```python
from build123d import *

# Parameters (mm, degrees)
SKETCH1_W                      = 55
SKETCH1_H                      = 55
BOSS_EXTRUDE1_DEPTH            = 6.35
SKETCH2_W                      = 11.25
SKETCH2_H                      = 11.25
CUT_EXTRUDE1_DEPTH             = 40.405868852
SKETCH3_W                      = 14
SKETCH3_H                      = 8.5
CUT_EXTRUDE2_DEPTH             = 2
CBORE_FOR_M2_SHCS2_D           = 2.4
CBORE_FOR_M2_SHCS2_CBORE_D     = 4.4
CBORE_FOR_M2_SHCS2_CBORE_DEPTH = 2
SKETCH6_R                      = 4
BOSS_EXTRUDE2_DEPTH            = 9.5
CBORE_FOR_M2_SHCS1_D           = 2.4
CBORE_FOR_M2_SHCS1_CBORE_D     = 4.4
CBORE_FOR_M2_SHCS1_CBORE_DEPTH = 2
SKETCH13_R                     = 3.025
CUT_EXTRUDE4_DEPTH             = 1
CHAMFER1_SIZE                  = 1.75
SKETCH16_W                     = 10
SKETCH16_H                     = 10
BOSS_EXTRUDE3_DEPTH            = 6.35
SKETCH17_R                     = 2.55
CUT_EXTRUDE6_DEPTH             = 50.129649907
FILLET1_R                      = 5
FILLET2_R                      = 1
SKETCH18_R                     = 3.025
CUT_EXTRUDE7_DEPTH             = 1
CUT_EXTRUDE8_DEPTH             = 0.6
CHAMFER2_SIZE                  = 1.5


with BuildPart() as part:
    # Sketch1 → Boss-Extrude1 (new body)
    with BuildSketch(Plane(origin=(0, 0, 0), x_dir=(1, 0, 0), z_dir=(0, 1, 0))):
        Rectangle(SKETCH1_W, SKETCH1_H)
    extrude(amount=BOSS_EXTRUDE1_DEPTH)

    # Sketch2 → Cut-Extrude1 (cut, through all)
    with BuildSketch(Plane(origin=(0, 6.35, 0), x_dir=(1, 0, 0), z_dir=(0, 1, 0))):
        Rectangle(SKETCH2_W, SKETCH2_H)
    extrude(amount=-CUT_EXTRUDE1_DEPTH, mode=Mode.SUBTRACT)

    # Sketch3 → Cut-Extrude2 (cut)
    with BuildSketch(Plane(origin=(0, 6.35, 0), x_dir=(1, 0, 0), z_dir=(0, 1, 0))):
        with Locations((0, -9.875)):
            Rectangle(SKETCH3_W, SKETCH3_H)
    extrude(amount=-CUT_EXTRUDE2_DEPTH, mode=Mode.SUBTRACT)

    # CBORE for M2 SHCS2 (through all)
    with Locations(Plane.XZ):
        with Locations((10.5, -0.1), (10.5, 12.4), (-10.5, 12.4), (-10.5, -0.1)):
            CounterBoreHole(CBORE_FOR_M2_SHCS2_D / 2, CBORE_FOR_M2_SHCS2_CBORE_D / 2, CBORE_FOR_M2_SHCS2_CBORE_DEPTH)

    # Sketch6 → Boss-Extrude2 (add)
    with BuildSketch(Plane(origin=(0, 6.35, 0), x_dir=(1, 0, 0), z_dir=(0, 1, 0))):
        with Locations(Location((-20, 20, 0), (0, 0, 270))):
            Circle(SKETCH6_R)
        with Locations(Location((20, 20, 0), (0, 0, 270))):
            Circle(SKETCH6_R)
        with Locations(Location((20, -20, 0), (0, 0, 270))):
            Circle(SKETCH6_R)
        with Locations(Location((-20, -20, 0), (0, 0, 270))):
            Circle(SKETCH6_R)
    extrude(amount=BOSS_EXTRUDE2_DEPTH)

    # CBORE for M2 SHCS1 (through all)
    with Locations(Plane.XZ):
        with Locations((-20, -20), (-20, 20), (20, 20), (20, -20)):
            CounterBoreHole(CBORE_FOR_M2_SHCS1_D / 2, CBORE_FOR_M2_SHCS1_CBORE_D / 2, CBORE_FOR_M2_SHCS1_CBORE_DEPTH)

    # Sketch13 → Cut-Extrude4 (cut)
    with BuildSketch(Plane(origin=(0, 6.35, 0), x_dir=(1, 0, 0), z_dir=(0, 1, 0))):
        with Locations(Location((-10.5, -12.4, 0), (0, 0, 270))):
            Circle(SKETCH13_R)
        with Locations(Location((-10.5, 0.1, 0), (0, 0, 270))):
            Circle(SKETCH13_R)
        with Locations(Location((10.5, -12.4, 0), (0, 0, 90))):
            Circle(SKETCH13_R)
        with Locations(Location((10.5, 0.1, 0), (0, 0, 90))):
            Circle(SKETCH13_R)
    extrude(amount=-CUT_EXTRUDE4_DEPTH, mode=Mode.SUBTRACT)

    # Chamfer1
    chamfer1_edges = [part.edges().sort_by_distance(p)[0] for p in [
        (5.625, 0, 0),
        (0, 0, 5.625),
        (-5.625, 0, 0),
        (0, 0, -5.625),
    ]]
    chamfer(chamfer1_edges, length=CHAMFER1_SIZE)

    # Sketch16 → Boss-Extrude3 (add)
    with BuildSketch(Plane.XZ):
        with Locations((32.5, 0)):
            Rectangle(SKETCH16_W, SKETCH16_H)
        with Locations((-32.5, 0)):
            Rectangle(SKETCH16_W, SKETCH16_H)
    extrude(amount=-BOSS_EXTRUDE3_DEPTH)

    # Sketch17 → Cut-Extrude6 (cut, through all)
    with BuildSketch(Plane.XZ):
        with Locations(Location((32.5, 0, 0), (0, 0, 270))):
            Circle(SKETCH17_R)
        with Locations(Location((-32.5, 0, 0), (0, 0, 270))):
            Circle(SKETCH17_R)
    extrude(amount=-CUT_EXTRUDE6_DEPTH, mode=Mode.SUBTRACT)

    # Fillet1
    fillet1_edges = [part.edges().sort_by_distance(p)[0] for p in [
        (27.5, 3.175, 5),
        (27.5, 3.175, -5),
        (-27.5, 3.175, -5),
        (-27.5, 3.175, 5),
        (27.5, 3.175, 27.5),
        (-27.5, 3.175, 27.5),
        (-27.5, 3.175, -27.5),
        (27.5, 3.175, -27.5),
    ]]
    fillet(fillet1_edges, radius=FILLET1_R)

    # Fillet2
    fillet2_edges = [part.edges().sort_by_distance(p)[0] for p in [
        (37.5, 3.175, -5),
        (37.5, 3.175, 5),
        (-37.5, 3.175, 5),
        (-37.5, 3.175, -5),
    ]]
    fillet(fillet2_edges, radius=FILLET2_R)

    # Sketch18 → Cut-Extrude7 (cut)
    with BuildSketch(Plane(origin=(0, 15.85, 0), x_dir=(1, 0, 0), z_dir=(0, 1, 0))):
        with Locations(Location((-20, 20, 0), (0, 0, 270))):
            Circle(SKETCH18_R)
        with Locations(Location((-20, -20, 0), (0, 0, 270))):
            Circle(SKETCH18_R)
        with Locations(Location((20, 20, 0), (0, 0, 270))):
            Circle(SKETCH18_R)
        with Locations(Location((20, -20, 0), (0, 0, 270))):
            Circle(SKETCH18_R)
    extrude(amount=-CUT_EXTRUDE7_DEPTH, mode=Mode.SUBTRACT)

    # Sketch19 → Cut-Extrude8 (cut)
    with BuildSketch(Plane(origin=(0, 6.35, 0), x_dir=(1, 0, 0), z_dir=(0, 1, 0))):
        Polygon((-2.301535791, 15.658119658), (-3.093589744, 15.658119658), (-3.093589744, 18.426068376), (-3.473504274, 18.426068376), (-3.473504274, 19.131623932), (-3.093589744, 19.131623932), (-3.093589744, 20), (-2.333760684, 20), (-2.333760684, 19.131623932), (-0.542735043, 19.131623932), (-0.542735043, 18.362466613), align=None)
        Polygon((-2.333760684, 18.426068376), (-2.333760684, 16.985276442), (-1.396694712, 18.426068376), align=None, mode=Mode.SUBTRACT)
        Polygon((3.55491453, 15.766666667), (2.743356036, 15.766666667), (1.65534188, 18.773758013), (0.564783654, 15.766666667), (-0.244230769, 15.766666667), (1.290691774, 20), (2.022536058, 20), align=None)
    extrude(amount=-CUT_EXTRUDE8_DEPTH, mode=Mode.SUBTRACT)

    # Chamfer2
    chamfer2_edges = [part.edges().sort_by_distance(p)[0] for p in [
        (-20, 6.35, -24),
        (20, 6.35, -24),
        (20, 6.35, 16),
        (-20, 6.35, 16),
    ]]
    chamfer(chamfer2_edges, length=CHAMFER2_SIZE)


solid = part.part
```
Verification items for the finished model (mm, model axes). A direction names the side the tool comes from. Round coordinates to 2 decimals unless told otherwise and drop trailing zeros. Write each loop counter-clockwise with the first axis right and the second up, starting at its lowest first coordinate (ties: lowest second). Pieces come first, ordered by that corner, then holes. Notation, with made-up numbers: (-28.75, 21.5) -> (-2.75, 21.5) arc R5 ccw to (-2.75, 27.5) -> close; hole circle Ø2 at (6, 75.5). An arc over 180 degrees is marked (long way). Write each question's results on one line, items separated by ' | '.
Q1. Sectioned sample at B-B, the plane z = 12.4. Give the number of separate pieces and of enclosed holes in the cut face, and give its area (3 significant figures).
Derived:
separate pieces: 3 | enclosed holes: 0 | area: 275 mm²
Q2. Sectioned sample at C-C, the plane x = -31. Record the boundary of the cut face in (y, z), and give its area (3 significant figures).
Derived:
outline: (0, -5.23) -> (6.35, -5.23) -> (6.35, -2.06) -> (0, -2.06) -> close; (0, 2.06) -> (6.35, 2.06) -> (6.35, 5.23) -> (0, 5.23) -> close | area: 40.2 mm²
Q3. Draft check along X on faces 1 (the face through (20.26, 8.51, -21.17)), 2 (the face through (-29, 3.22, -6.43)), 3 (the face through (27.5, 3, 16)). Enter one of: released by +X, released by -X, zero draft, split by the parting line, or undercut.
Derived:
face 1: undercut | face 2: released by -X | face 3: released by +X
Q4. Thickness scan on probe 1 along Z at (x, y) = (20, 1.05); probe 2 along X at (y, z) = (1.5, 21.5); probe 3 along Z at (x, y) = (-9, 5.5). Record the ranges inside material, lowest first.
Derived:
probe 1: z = -27.5 to -22.2, -17.8 to 17.8, 22.2 to 27.5 | probe 2: x = -27.5 to -21.61, -18.39 to 18.39, 21.61 to 27.5 | probe 3: z = -27.5 to -2.73, 2.53 to 9.77, 15.03 to 27.5
Q5. Sectioned sample at A-A, the plane y = 12. Record the boundary of the cut face in (x, z), and give its area (3 significant figures).
Derived:
outline: circle Ø8 at (-20, -20); circle Ø8 at (-20, 20); circle Ø8 at (20, -20); circle Ø8 at (20, 20); hole circle Ø2.4 at (-20, -20); hole circle Ø2.4 at (-20, 20); hole circle Ø2.4 at (20, -20); hole circle Ø2.4 at (20, 20) | area: 183 mm²
Q6. Access from +Z, -Z, +X, -X, +Y, -Y to the whole of each face (thin tool, end or side, straight path). Record for faces 4 (the face through (0, 3, 5.625)), 5 (the face through (27.5, 3, -16)), 6 (the face through (-27.5, 3, -16)).
Derived:
face 4: +Y, -Y | face 5: -Z, +X, +Y, -Y | face 6: -Z, -X, +Y, -Y
Q7. Go/stop test with flat-tipped pins: pin 1 Ø6 at (y, z) = (7, 21) entering from -X; pin 2 Ø1 at (y, z) = (5, 8) entering from -X; pin 3 Ø12 at (x, z) = (-11, -14) entering from +Y; pin 4 Ø1.9 at (x, z) = (10.5, 12.4) entering from -Y. Record where each tip stops, or that it passes through.
Derived:
pin 1: stops at x = -27.5 | pin 2: stops at x = -28.17 | pin 3: stops at y = 7.03 | pin 4: passes through
